```python
from build123d import *

# Parameters (mm, degrees)
EXTRUDE1_DEPTH      = 150
EXTRUDE1_DEPTH_BACK = 150


with BuildPart() as part:
    # Sketch1 → Extrude1 (new body, two sides)
    with BuildSketch(Plane.XY) as extrude1_sk:
        with BuildLine():
            Line((-500, 27), (500, 27))
            ThreePointArc((500, 27), (527, 0), (500, -27))
            Line((500, -27), (-500, -27))
            ThreePointArc((-500, -27), (-527, 0), (-500, 27))
        make_face()
        with BuildLine():
            Line((-500, 25), (500, 25))
            ThreePointArc((500, 25), (525, 0), (500, -25))
            Line((500, -25), (-500, -25))
            ThreePointArc((-500, -25), (-525, 0), (-500, 25))
        make_face(mode=Mode.SUBTRACT)
    extrude(amount=EXTRUDE1_DEPTH)
    extrude(extrude1_sk.sketch, amount=-EXTRUDE1_DEPTH_BACK)


solid = part.part
```
Part model, mm, in its own coordinate system. A direction names the side the tool comes from. Round coordinates to 2 decimals unless told otherwise and drop trailing zeros. Loops run counter-clockwise (first coordinate to the right, second up) from the corner with the lowest first, then second, coordinate; pieces in that order, holes last. Notation, with made-up numbers: (25, 20) -> (56, 20) arc R18 ccw to (56, 48) -> close; hole circle Ø4 at (-20, 44). An arc over 180 degrees is marked (long way). Use a Markdown table: item, result.
1) Drop flat-ended pins along their axis: pin 1 Ø1.5 at (y, z) = (10.5, 103) entering from -X; pin 2 Ø10 at (y, z) = (13, -116) entering from +X. Give the stop position or say it passes through.
The answers:
| item | result |
|---|---|
| pin 1 | stops at x = -525.18 |
| pin 2 | stops at x = 525.79 |
2) Tool access for faces 1 (the cylindrical face through (524.994, 0.55, 2.1)), 2 (the cylindrical face through (-526.993, -0.594, 2.1)): list every direction of +Z, -Z, +X, -X, +Y, -Y with a clear straight run to the whole face (end or side of a thin tool).
The answers:
| item | result |
|---|---|
| face 1 | +Z, -Z |
| face 2 | +Z, -Z, -X |
3) Cut at B-B, the plane x = -322.5. List the corners of the cut face in (y, z), and give its area (3 significant figures).
The answers:
| item | result |
|---|---|
| outline | (-27, -150) -> (-25, -150) -> (-25, 150) -> (-27, 150) -> close; (25, -150) -> (27, -150) -> (27, 150) -> (25, 150) -> close |
| area | 1,200 mm2 |
4) Probe line 1 (Y direction, x = -74.5, z = -127.5); line 2 (X direction, y = 8, z = -54.5); line 3 (X direction, y = -22, z = 29). List the from-to ranges inside material, lowest first. Write a range as [from, to].
The answers:
| item | result |
|---|---|
| line 1 | y = [-27, -25], [25, 27] |
| line 2 | x = [-525.79, -523.69], [523.69, 525.79] |
| line 3 | x = [-515.65, -511.87], [511.87, 515.65] |
5) Pull direction Y, two halves, no side cores. Call faces 3 (the flat face through (7, -25, 2)), 4 (the flat face through (-7, 27, 2)), 5 (the flat face through (2, 26, 150)): pulls with the +Y half, pulls with the -Y half, needs draft (parallel to the pull), parting line crosses it, or undercut.
The answers:
| item | result |
|---|---|
| face 3 | undercut |
| face 4 | pulls with the +Y half |
| face 5 | needs draft |
6) Cut at A-A, the plane z = -32.5. List the corners of the cut face in (x, y), and give its area (3 significant figures).
The answers:
| item | result |
|---|---|
| outline | (-500, -27) -> (500, -27) arc R27 ccw to (500, 27) -> (-500, 27) arc R27 ccw to start; hole (-500, -25) -> (500, -25) arc R25 ccw to (500, 25) -> (-500, 25) arc R25 ccw to start |
| area | 4,330 mm2 |
7) Cut at C-C, the plane y = 0. List the corners of the cut face in (x, z), and give its area (3 significant figures).
The answers:
| item | result |
|---|---|
| outline | (-527, -150) -> (-525, -150) -> (-525, 150) -> (-527, 150) -> close; (525, -150) -> (527, -150) -> (527, 150) -> (525, 150) -> close |
| area | 1,200 mm2 |
